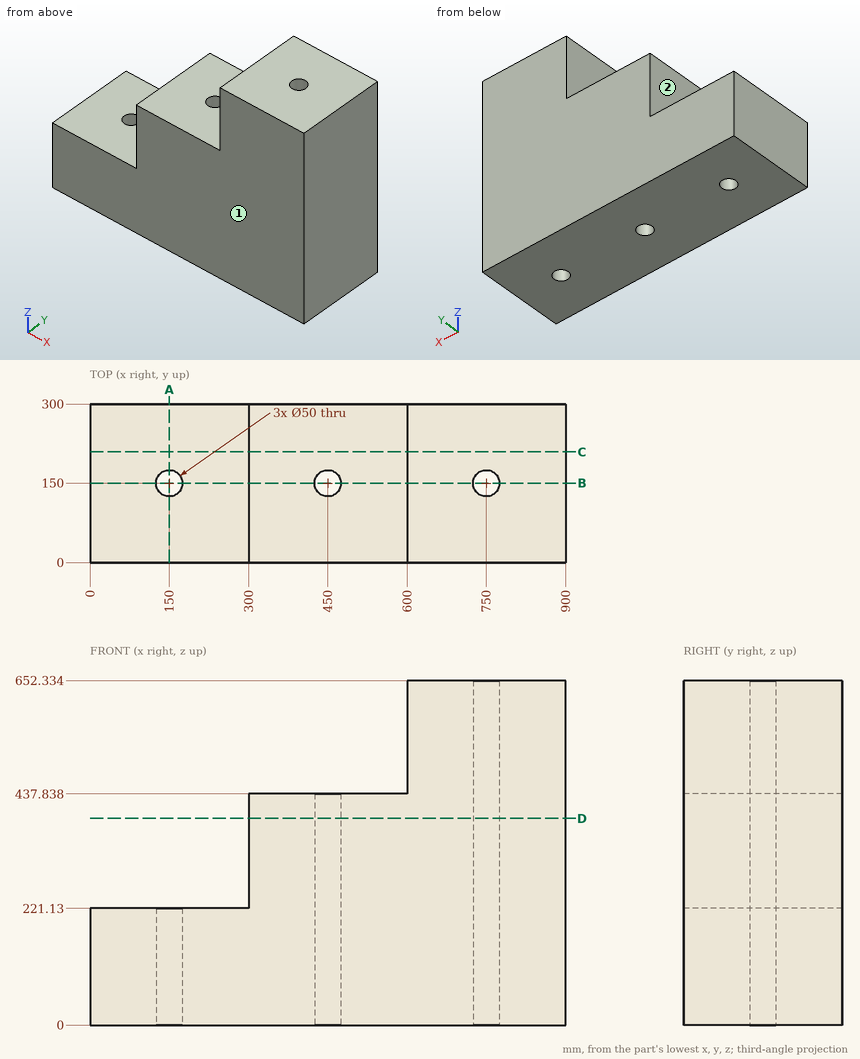
The drawing under review shows one solid part. Ordinate dimensions are in mm from its lowest x, y, z. A direction names the side the tool comes from. Round coordinates to 2 decimals unless told otherwise and drop trailing zeros. Loops run counter-clockwise (first coordinate to the right, second up) from the corner with the lowest first, then second, coordinate; pieces in that order, holes last. Notation, with made-up numbers: (86.5, 80) - (108.5, 80) arc R11 cw to (108.5, 94) - close; hole circle Ø9 at (-24.5, 50.5). An arc over 180 degrees is marked (long way). Put each result on its own line as item: value. Start each with the question number.
1. Consider section A-A on x = 150. State the section outline as (y, z) points, plus the area to 3 significant figures.
2. Consider section D-D on z = 391.5. State the section outline as (x, y) points.
3. Consider section C-C on y = 209.5. State the section outline as (x, z) points.
4. For the marked faces 1 and 2, list the 3-axis set-ups (+Z, -Z, +X, -X, +Y, -Y) from which the entire face can be reached by the end or side of a thin tool; tool diameter is ignored.
5. Insertion check: P1, Ø1.5, axis at y = 62.5, z = 161.5, coming from the -X side; P2, Ø12, axis at y = 128, z = 496, coming from the -X side; P3, Ø1, axis at x = 328.5, y = 200, coming from the +Z side; P4, Ø1, axis at y = 265.5, z = 409.5, coming from the -X side. Each pin has a flat end and moves straight along its axis. Give the tip position at first contact, or say it passes through.
6. For probe 1 along Y at (x, z) = (150, 101); probe 2 along Z at (x, y) = (447, 206.5); probe 3 along X at (y, z) = (60.5, 522), list the stretches that pass through material, from the lowest coordinate up. Write a range as [from, to].
7. Consider section B-B on y = 150. State the section outline as (x, z) points, plus the area to 3 significant figures.
Result sheet:
1. outline: (0, 0) - (125, 0) - (125, 221.13) - (0, 221.13) - close; (175, 0) - (300, 0) - (300, 221.13) - (175, 221.13) - close
1. area: 55,300 mm^2
2. outline: (300, 0) - (900, 0) - (900, 300) - (300, 300) - close; hole circle Ø50 at (450, 150); hole circle Ø50 at (750, 150)
3. outline: (0, 0) - (900, 0) - (900, 652.33) - (600, 652.33) - (600, 437.84) - (300, 437.84) - (300, 221.13) - (0, 221.13) - close
4. face 1: +Z, -Z, +X, -X, -Y
4. face 2: +Z, -X, +Y, -Y
5. P1: x = 0
5. P2: x = 600
5. P3: z = 437.84
5. P4: x = 300
6. probe 1: [0, 125], [175, 300]
6. probe 2: [0, 437.84]
6. probe 3: [600, 900]
7. outline: (0, 0) - (125, 0) - (125, 221.13) - (0, 221.13) - close; (175, 0) - (425, 0) - (425, 437.84) - (300, 437.84) - (300, 221.13) - (175, 221.13) - close; (475, 0) - (725, 0) - (725, 652.33) - (600, 652.33) - (600, 437.84) - (475, 437.84) - close; (775, 0) - (900, 0) - (900, 652.33) - (775, 652.33) - close
7. area: 328,000 mm^2
